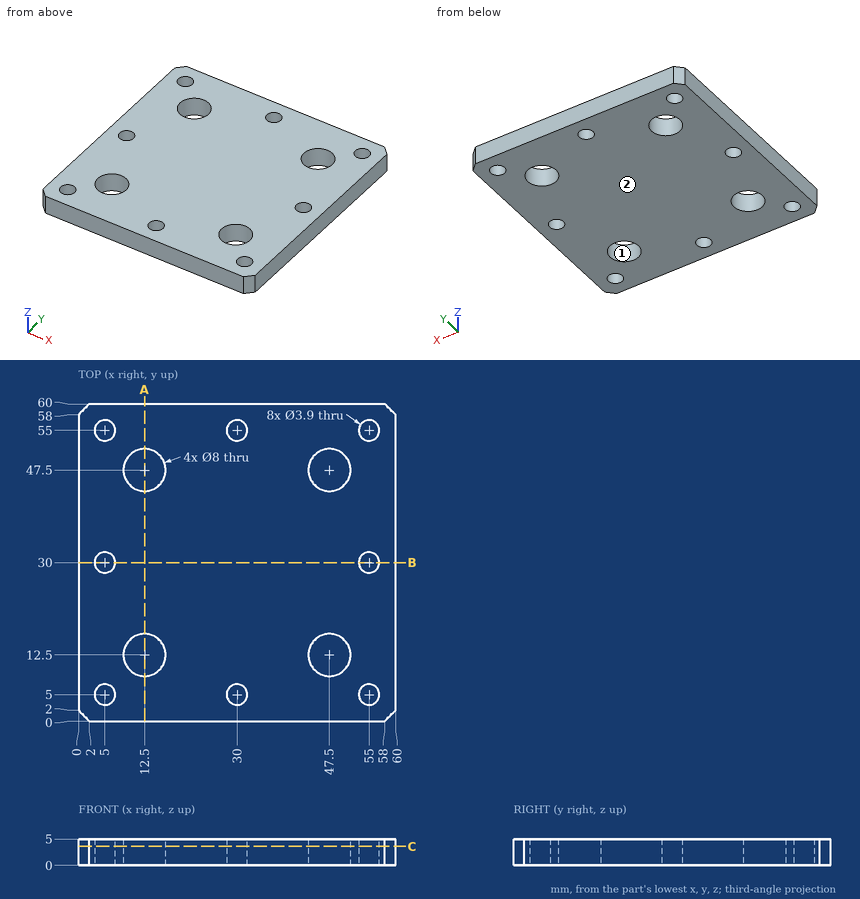
Design review of the part shown in the three views and the two pictorial views. Dimensions are in mm from the part's minimum x, y and z. Coordinates: 2 decimals unless noted, no trailing zeros. Write each loop counter-clockwise with the first axis right and the second up, starting at its lowest first coordinate (ties: lowest second). Pieces come first, ordered by that corner, then holes. Notation, with made-up numbers: (-16.75, 49) -> (13.25, 49) arc R16 cw to (13.25, 79) -> close; hole circle Ø3 at (83, 16). An arc over 180 degrees is marked (long way). Answer in a Markdown table with one row per item.
1. We need section B-B, the plane y = 30. State the section outline as (x, z) points.
Answers below:
| item | result |
|---|---|
| outline | (0, 0) -> (3.05, 0) -> (3.05, 5) -> (0, 5) -> close; (6.95, 0) -> (53.05, 0) -> (53.05, 5) -> (6.95, 5) -> close; (56.95, 0) -> (60, 0) -> (60, 5) -> (56.95, 5) -> close |
2. Draft analysis for pull direction Y (two halves, no side actions). For the marked faces 1 and 2, state which applies: +Y half, -Y half, draft (parallel to the pull), parting line (faces both ways), or undercut.
Answers below:
| item | result |
|---|---|
| face 1 | undercut |
| face 2 | draft |
3. We need section A-A, the plane x = 12.5. State the section outline as (y, z) points, and give its area (3 significant figures).
Answers below:
| item | result |
|---|---|
| outline | (0, 0) -> (8.5, 0) -> (8.5, 5) -> (0, 5) -> close; (16.5, 0) -> (43.5, 0) -> (43.5, 5) -> (16.5, 5) -> close; (51.5, 0) -> (60, 0) -> (60, 5) -> (51.5, 5) -> close |
| area | 220 mm^2 |
4. We need section C-C, the plane z = 3.6. Give the number of separate pieces and of enclosed holes in the cut face, and give its area (3 significant figures).
Answers below:
| item | result |
|---|---|
| separate pieces | 1 |
| enclosed holes | 12 |
| area | 3,300 mm^2 |
5. Clearance check with a flat-ended pin moving along its axis: pin 1 Ø6.5 at (x, y) = (12.5, 47.5) entering from -Z. State where the tip first meets the part, or that it passes through.
Answers below:
| item | result |
|---|---|
| pin 1 | passes through |
6. Wall thickness on probe 1 along Y at (x, z) = (12.5, 3.65); probe 2 along X at (y, z) = (54.5, 2.4); probe 3 along X at (y, z) = (29, 2.95): over which ranges is each line inside the solid? List them lowest first. Write a range as [from, to].
Answers below:
| item | result |
|---|---|
| probe 1 | y = [0, 8.5], [16.5, 43.5], [51.5, 60] |
| probe 2 | x = [0, 3.12], [6.88, 28.12], [31.88, 53.12], [56.88, 60] |
| probe 3 | x = [0, 3.33], [6.67, 53.33], [56.67, 60] |
